from build123d import *

# Parameters (mm, degrees)
BOSS_EXTRUDE2_DEPTH = 50
SKETCH3_R           = 2.5
CUT_EXTRUDE2_DEPTH  = 50


with BuildPart() as part:
    # Sketch1 → Boss-Extrude2 (new body)
    with BuildSketch(Plane.XY):
        with BuildLine():
            Line((-50, 0), (-14.803348106, 0))
            ThreePointArc((-14.803348106, 0), (0, 33.448452879), (14.803348106, 0))
            Line((14.803348106, 0), (50, 0))
            Line((50, 0), (50, -2))
            Line((50, -2), (9.238252196, -2))
            ThreePointArc((9.238252196, -2), (0, 31.448452879), (-9.238252196, -2))
            Line((-9.238252196, -2), (-50, -2))
            Line((-50, -2), (-50, 0))
        make_face()
    extrude(amount=BOSS_EXTRUDE2_DEPTH)

    # Sketch3 → Cut-Extrude2 (cut)
    with BuildSketch(Plane(origin=(0, 0, 0), x_dir=(1, 0, 0), z_dir=(0, 1, 0))):
        with Locations((35, -10)):
            Circle(SKETCH3_R)
        with Locations((35, -40)):
            Circle(SKETCH3_R)
        with Locations((-35, -40)):
            Circle(SKETCH3_R)
        with Locations((-35, -10)):
            Circle(SKETCH3_R)
    extrude(amount=-CUT_EXTRUDE2_DEPTH, mode=Mode.SUBTRACT)


solid = part.part
Can you work these out from the model? Positions are in its coordinate system, mm. Give positions to 0.01 mm unless a question says otherwise; leave off trailing zeros. Order: outer loops, then holes, each group sorted by start corner. A loop starts at its lowest first (then second) coordinate and runs counter-clockwise, first axis right, second up. Notation, with made-up numbers: M -3.75,74.25 L 19.25,74.25 A25 cw 19.25,110.25 Z; hole C 26.25,-8 d2. An arc over 180 degrees is marked long. Use a Markdown table: item, result. Add a question column.
Item 1: Suppose I cut it at A-A (x = 35). List the corners of the cut face in (y, z) for me.
Item 2: Suppose I cut it at D-D (z = 4). List the corners of the cut face in (x, y) for me.
Item 3: Suppose I cut it at B-B (z = 39). List the corners of the cut face in (x, y) for me, then the cut area to 3 significant figures.
Item 4: We'd pull the mould along Z, two halves only. Please class faces 1 (the cylindrical face through (37.31, -0.99, 40.96)), 2 (the flat face through (30, -2, 25)), 3 (the flat face through (-11, -1, 50)), 4 (the flat face through (-11, -1, 0)): +Z half, -Z half, draft (parallel to the pull), parting line (faces both ways), or undercut.
Item 5: Will these pins go through, and if not, where does the flat tip stop? pin 1 (6.5 mm diameter, centred on x = -35, z = 10, fed in from +Y); pin 2 (1.5 mm diameter, centred on y = 11, z = 29, fed in from -X); pin 3 (2 mm diameter, centred on y = 6, z = 5.5, fed in from +X).
Item 6: If I drill on L1, parallel to Z at x = 35, y = -0.35; L2, parallel to X at y = 13, z = 26.5; L3, parallel to Y at x = -15, z = 43, over which ranges is the centre line in solid material (lowest first)? Write a range as [from, to].
Item 7: Suppose I cut it at C-C (y = 2). List the corners of the cut face in (x, z) for me.
Answer sheet:
| question | item | result |
|---|---|---|
| 1 | outline | M -2,0 L 0,0 L 0,7.5 L -2,7.5 Z; M -2,12.5 L 0,12.5 L 0,37.5 L -2,37.5 Z; M -2,42.5 L 0,42.5 L 0,50 L -2,50 Z |
| 2 | outline | M -50,-2 L -9.24,-2 A18 cw long 9.24,-2 L 50,-2 L 50,0 L 14.8,0 A20 ccw long -14.8,0 L -50,0 Z |
| 3 | outline | M -50,-2 L -37.29,-2 L -37.29,0 L -50,0 Z; M -32.71,-2 L -9.24,-2 A18 cw long 9.24,-2 L 32.71,-2 L 32.71,0 L 14.8,0 A20 ccw long -14.8,0 L -32.71,0 Z; M 37.29,-2 L 50,-2 L 50,0 L 37.29,0 Z |
| 3 | area | 318 mm² |
| 4 | face 1 | undercut |
| 4 | face 2 | draft |
| 4 | face 3 | +Z half |
| 4 | face 4 | -Z half |
| 5 | pin 1 | stops at y = 0 |
| 5 | pin 2 | stops at x = -19.93 |
| 5 | pin 3 | stops at x = 18.93 |
| 6 | L1 | z = [0, 7.5], [12.5, 37.5], [42.5, 50] |
| 6 | L2 | x = [-19.99, -17.99], [17.99, 19.99] |
| 6 | L3 | y = [-2, 0], [0.22, 3.5], [23.4, 26.68] |
| 7 | outline | M -16.4,0 L -13.89,0 L -13.89,50 L -16.4,50 Z; M 13.89,0 L 16.4,0 L 16.4,50 L 13.89,50 Z |
